Part model, mm, in its own coordinate system. A direction names the side the tool comes from. Give positions to 0.01 mm unless a question says otherwise; leave off trailing zeros. Write each loop counter-clockwise with the first axis right and the second up, starting at its lowest first coordinate (ties: lowest second). Pieces come first, ordered by that corner, then holes.
from build123d import *

# Parameters (mm, degrees)
SKETCH1_R               = 3.475
BOSS_EXTRUDE1_DEPTH     = 12
CUT_EXTRUDE3_START      = -29.3
CUT_EXTRUDE3_OUTLINE_R  = 2.1
CUT_EXTRUDE3_DEPTH      = 29.3
SKETCH3_W               = 2.25
SKETCH3_H               = 7.15
CUT_EXTRUDE4_DEPTH      = 9.5
CUT_EXTRUDE6_DEPTH      = 7.2
CUT_EXTRUDE6_DEPTH_BACK = 11.2
SKETCH4_R               = 2.125


# Read off the part's stored shape, not the designer's step: Cut-Extrude3
with BuildPart() as part:
    # Sketch1 → Boss-Extrude1 (new body)
    with BuildSketch(Plane.XY):
        with BuildLine():
            Line((-14.65, 20), (-14.65, -5.35))
            ThreePointArc((-14.65, -5.35), (0, -20), (14.65, -5.35))
            Line((14.65, -5.35), (14.65, 20))
            Line((14.65, 20), (12.65, 20))
            Line((12.65, 20), (12.65, 7.005))
            ThreePointArc((12.65, 7.005), (0, -5.645), (-12.65, 7.005))
            Line((-12.65, 7.005), (-12.65, 20))
            Line((-12.65, 20), (-14.65, 20))
        make_face()
        with Locations((0, -12.825)):
            Circle(SKETCH1_R, mode=Mode.SUBTRACT)
    extrude(amount=BOSS_EXTRUDE1_DEPTH)

    # Cut-Extrude3 outline → Cut-Extrude3 (cut)
    with BuildSketch(Plane.ZY.offset(14.65).offset(CUT_EXTRUDE3_START)):
        with BuildLine():
            ThreePointArc((0, 14), (1.757359313, 18.242640687), (6, 20))
            Line((6, 20), (0, 20))
            Line((0, 20), (0, 14))
        make_face()
        with BuildLine():
            ThreePointArc((6, 20), (10.242640687, 18.242640687), (12, 14))
            Line((12, 14), (12, 20))
            Line((12, 20), (6, 20))
        make_face()
        with Locations((6, 14)):
            Circle(CUT_EXTRUDE3_OUTLINE_R)
    extrude(amount=CUT_EXTRUDE3_DEPTH, mode=Mode.SUBTRACT)

    # Sketch3 → Cut-Extrude4 (cut)
    with BuildSketch(Plane.XY.offset(12)):
        with Locations((5.6, -12.825)):
            Rectangle(SKETCH3_W, SKETCH3_H)
    extrude(amount=-CUT_EXTRUDE4_DEPTH, mode=Mode.SUBTRACT)

    # Sketch4 → Cut-Extrude6 (cut, two sides: drawn at the far end of the back side and taken through both)
    with BuildSketch(Plane.ZY.offset(-6.725).offset(-CUT_EXTRUDE6_DEPTH_BACK)):
        with Locations(Location((6.075, -12.825, 0), (0, 0, 90))):
            Circle(SKETCH4_R)
    extrude(amount=CUT_EXTRUDE6_DEPTH + CUT_EXTRUDE6_DEPTH_BACK, mode=Mode.SUBTRACT)


solid = part.part
1) Saw through at A-A (y = 7.5). Write the cut outline in (x, z).
Check result:
outline: (-14.65, 0) - (-12.65, 0) - (-12.65, 12) - (-14.65, 12) - close; (12.65, 0) - (14.65, 0) - (14.65, 12) - (12.65, 12) - close
2) Drill centre lines: L1, parallel to Z at x = 7.5, y = -13; L2, parallel to Z at x = 13.7, y = 14; L3, parallel to X at y = 17.5, z = 2. Where is each one in solid material? Low to high.
Check result:
L1: z = 0 to 3.96, 8.19 to 12
L2: z = 0 to 3.9, 8.1 to 12
L3: x = -14.65 to -12.65, 12.65 to 14.65
3) Mould opens along Z. For faces 4 (the flat face through (6, -9.25, 7)), 5 (the cylindrical face through (9.462, -10.862, 6.889)), 6 (the flat face through (0, -7, 12)) say: +Z half, -Z half, draft (parallel to the pull), parting line (faces both ways), or undercut.
Check result:
face 4: draft
face 5: undercut
face 6: +Z half
4) Saw through at D-D (z = 2). Write the cut outline in (x, y) (3 decimals), and give its area (3 significant figures).
Check result:
outline: (-14.65, -5.35) arc R14.65 ccw to (14.65, -5.35) - (14.65, 18.472) - (12.65, 18.472) - (12.65, 7.005) arc R12.65 cw to (-12.65, 7.005) - (-12.65, 18.472) - (-14.65, 18.472) - close; hole circle Ø6.95 at (0, -12.825)
area: 456 mm2
5) Saw through at C-C (x = -2.5). Write the cut outline in (y, z), and give its area (3 significant figures).
Check result:
outline: (-19.79, 0) - (-15.24, 0) - (-15.24, 12) - (-19.79, 12) - close; (-10.41, 0) - (-5.4, 0) - (-5.4, 12) - (-10.41, 12) - close
area: 115 mm2
6) 3-axis set-ups, long thin cutter, end or side, ignore diameter. For faces 1 (the flat face through (12.65, 12.1, 4.6)), 2 (the flat face through (6.725, -12.9, 8.4)), 3 (the cylindrical face through (3.82, -14.51, 7.37)): which of +Z, -Z, +X, -X, +Y, -Y reach the whole face in a straight line?
Check result:
face 1: +Z, -Z, +Y
face 2: +Z
face 3: +X
7) Saw through at B-B (z = 7). Write the cut outline in (x, y) (3 decimals), and give its area (3 significant figures).
Check result:
outline: (-14.65, -5.35) arc R14.65 ccw to (11.247, -14.738) - (6.725, -14.738) - (6.725, -16.4) - (4.475, -16.4) - (4.475, -14.738) - (2.901, -14.738) arc R3.475 cw (long way) to (2.901, -10.912) - (4.475, -10.912) - (4.475, -9.25) - (6.725, -9.25) - (6.725, -10.912) - (13.553, -10.912) arc R14.65 ccw to (14.65, -5.35) - (14.65, 12.153) - (12.65, 12.153) - (12.65, 7.005) arc R12.65 cw to (-12.65, 7.005) - (-12.65, 12.153) - (-14.65, 12.153) - close; (-14.65, 15.847) - (-12.65, 15.847) - (-12.65, 19.916) - (-14.65, 19.916) - close; (12.65, 15.847) - (14.65, 15.847) - (14.65, 19.916) - (12.65, 19.916) - close
area: 404 mm2
8) Flat gauge pins, fed straight in: P1, Ø5.5, axis at y = -12.825, z = 6.075, coming from the +X side; P2, Ø1.8, axis at x = 5, z = 8, coming from the +Y side; P3, Ø3.5, axis at y = -12.5, z = 5.5, coming from the -X side. Where does each tip first touch, or does it go through?
Check result:
P1: stops at x = 13.87
P2: stops at y = -4.18
P3: stops at x = -13.62
